from build123d import *

# Parameters (mm, degrees)
SKETCH2_W           = 119.38
SKETCH2_H           = 92.71
SKETCH2_W_2         = 109.728
SKETCH2_H_2         = 83.058
BOSS_EXTRUDE1_DEPTH = 25.4
FILLET1_R           = 2.54


with BuildPart() as part:
    # Sketch2 → Boss-Extrude1 (new body)
    with BuildSketch(Plane(origin=(0, 0, 0), x_dir=(1, 0, 0), z_dir=(0, 1, 0))):
        with Locations((59.69, 46.355)):
            Rectangle(SKETCH2_W, SKETCH2_H)
        with Locations((59.69, 46.355)):
            Rectangle(SKETCH2_W_2, SKETCH2_H_2, mode=Mode.SUBTRACT)
    extrude(amount=BOSS_EXTRUDE1_DEPTH)

    # Fillet1
    fillet1_edges = [part.edges().sort_by_distance(p)[0] for p in [
        (0, 12.7, -92.71),
        (119.38, 12.7, -92.71),
        (119.38, 12.7, 0),
        (0, 12.7, 0),
    ]]
    fillet(fillet1_edges, radius=FILLET1_R)


solid = part.part
The model under review builds one solid part; all positions refer to its coordinate system, in mm. A direction names the side the tool comes from. Round coordinates to 2 decimals unless told otherwise and drop trailing zeros. Write each loop counter-clockwise with the first axis right and the second up, starting at its lowest first coordinate (ties: lowest second). Pieces come first, ordered by that corner, then holes. Notation, with made-up numbers: (15.5, 71) - (73.5, 71) arc R22 cw to (73.5, 80) - close; hole circle Ø11 at (69.5, 80.25). An arc over 180 degrees is marked (long way). One line per item, written item: value. Start each with the question number.
1. Machinability: for faces 4 (the face through (119.38, 13, -46)), 5 (the face through (59, 13, -87.884)), which of the approach directions +Z, -Z, +X, -X, +Y, -Y give a long, thin tool a straight path to every point of the face, cutting with its end or side? Answer none if there is none.
2. Consider section B-B on z = -69. Write out the cut boundary in (x, y).
3. Consider section A-A on x = 77. Write out the cut boundary in (y, z), and give its area (3 significant figures).
4. Consider section C-C on y = 21.5. Write out the cut boundary in (x, z), and give its area (3 significant figures).
5. The part is to be moulded in two halves that separate along X. For faces 1 (the face through (59, 13, -4.826)), 2 (the face through (55, 25.4, -2)), 3 (the face through (0.724, 12.878, -0.764)), say which applies: released by +X, released by -X, zero draft, split by the parting line, or undercut.
6. Clearance check with a flat-ended pin moving along its axis: P1, Ø12, axis at x = 67, z = -76, coming from the -Y side. State where the tip first meets the part, or that it passes through.
7. To check wall thickness, follow L1, parallel to Z at x = 104, y = 17; L2, parallel to X at y = 17.5, z = -53. State the ranges of each line that lie inside material, in increasing order. Write a range as from..to.
Checks:
1. face 4: +Z, -Z, +X, +Y, -Y
1. face 5: +Y, -Y
2. outline: (0, 0) - (4.83, 0) - (4.83, 25.4) - (0, 25.4) - close; (114.55, 0) - (119.38, 0) - (119.38, 25.4) - (114.55, 25.4) - close
3. outline: (0, -92.71) - (25.4, -92.71) - (25.4, -87.88) - (0, -87.88) - close; (0, -4.83) - (25.4, -4.83) - (25.4, 0) - (0, 0) - close
3. area: 245 mm^2
4. outline: (0, -90.17) arc R2.54 ccw to (2.54, -92.71) - (116.84, -92.71) arc R2.54 ccw to (119.38, -90.17) - (119.38, -2.54) arc R2.54 ccw to (116.84, 0) - (2.54, 0) arc R2.54 ccw to (0, -2.54) - close; hole (4.83, -87.88) - (114.55, -87.88) - (114.55, -4.83) - (4.83, -4.83) - close
4. area: 1,950 mm^2
5. face 1: undercut
5. face 2: zero draft
5. face 3: released by -X
6. P1: passes through
7. L1: z = -92.71..-87.88, -4.83..0
7. L2: x = 0..4.83, 114.55..119.38
